Source: three-view drawing plus pictorial views. Frame: mm from the lowest corner of the part. A direction names the side the tool comes from. Give positions to 0.01 mm unless a question says otherwise; leave off trailing zeros. Loops run counter-clockwise (first coordinate to the right, second up) from the corner with the lowest first, then second, coordinate; pieces in that order, holes last. Notation, with made-up numbers: (-16, 13) -> (39, 13) arc R20 cw to (39, 33) -> close; hole circle Ø1 at (11.25, 47.25). An arc over 180 degrees is marked (long way). Answer as a JSON object with one key per item and string values. Group by question number.
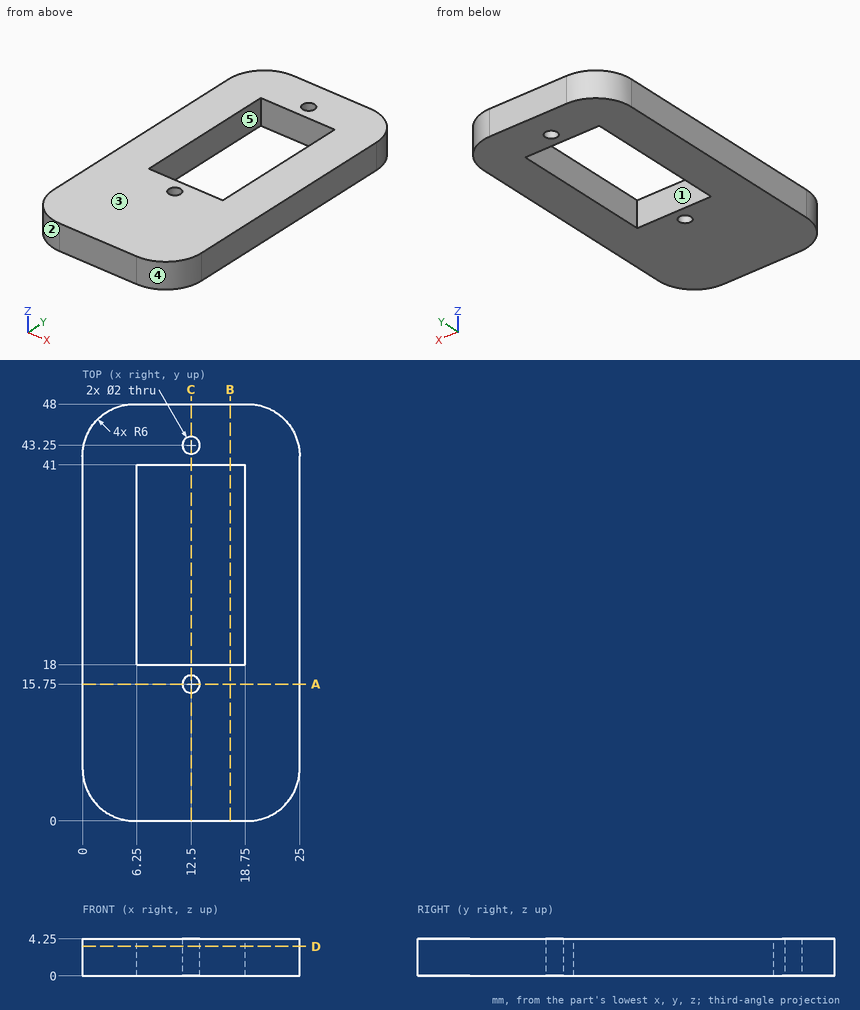
Q1. Ray query, probe 1 along Y at (x, z) = (12.5, 2.8); probe 2 along Y at (x, z) = (7.5, 2.1); probe 3 along X at (y, z) = (23.5, 1.8). Return the intervals inside material, ascending.
Q2. Set-up query: the marked faces 4 and 5. Return all of +Z, -Z, +X, -X, +Y, -Y with unobstructed straight access to the full face (end or side cutting, diameter ignored); none if empty.
Q3. Section A-A on y = 15.75. Return the cut outline in (x, z), then the cut area to 4 significant figures.
Q4. Section B-B on x = 17. Return the cut outline in (y, z).
Q5. Section C-C on x = 12.5. Return the cut outline in (y, z), then the cut area to 4 significant figures.
Q6. Section D-D on z = 3.4. Return the cut outline in (x, y), then the cut area to 3 significant figures.
Q7. Pull-direction query (Y, two-part tool) for the marked faces 1, 2 and 3; classes: +Y half, -Y half, draft (parallel to the pull), parting line (faces both ways), or undercut.
Numbers:
{
 "1": {"probe 1": "y = 0 to 14.75, 16.75 to 18, 41 to 42.25, 44.25 to 48", "probe 2": "y = 0 to 18, 41 to 48", "probe 3": "x = 0 to 6.25, 18.75 to 25"},
 "2": {"face 4": "+Z, -Z, +X, -Y", "face 5": "+Z, -Z"},
 "3": {"outline": "(0, 0) -> (11.5, 0) -> (11.5, 4.25) -> (0, 4.25) -> close; (13.5, 0) -> (25, 0) -> (25, 4.25) -> (13.5, 4.25) -> close", "area": "97.75 mm²"},
 "4": {"outline": "(0, 0) -> (18, 0) -> (18, 4.25) -> (0, 4.25) -> close; (41, 0) -> (48, 0) -> (48, 4.25) -> (41, 4.25) -> close"},
 "5": {"outline": "(0, 0) -> (14.75, 0) -> (14.75, 4.25) -> (0, 4.25) -> close; (16.75, 0) -> (18, 0) -> (18, 4.25) -> (16.75, 4.25) -> close; (41, 0) -> (42.25, 0) -> (42.25, 4.25) -> (41, 4.25) -> close; (44.25, 0) -> (48, 0) -> (48, 4.25) -> (44.25, 4.25) -> close", "area": "89.25 mm²"},
 "6": {"outline": "(0, 6) arc R6 ccw to (6, 0) -> (19, 0) arc R6 ccw to (25, 6) -> (25, 42) arc R6 ccw to (19, 48) -> (6, 48) arc R6 ccw to (0, 42) -> close; hole (6.25, 18) -> (18.75, 18) -> (18.75, 41) -> (6.25, 41) -> close; hole circle Ø2 at (12.5, 15.75); hole circle Ø2 at (12.5, 43.25)", "area": "875 mm²"},
 "7": {"face 1": "undercut", "face 2": "-Y half", "face 3": "draft"}
}
